Can you work these out from the model? Positions are in its coordinate system, mm. Round coordinates to 2 decimals unless told otherwise and drop trailing zeros. Order: outer loops, then holes, each group sorted by start corner. A loop starts at its lowest first (then second) coordinate and runs counter-clockwise, first axis right, second up. Notation, with made-up numbers: (17.5, 3.25) - (34.5, 3.25) arc R22 ccw to (34.5, 11.25) - close; hole circle Ø10 at (30, 70). An arc over 180 degrees is marked (long way). Write item = value, one per line.
from build123d import *

# Parameters (mm, degrees)
BOSS_EXTRUDE1_DEPTH = 2
SKETCH2_W           = 40
SKETCH2_H           = 13
BOSS_EXTRUDE2_DEPTH = 2.8


with BuildPart() as part:
    # Sketch1 → Boss-Extrude1 (new body)
    with BuildSketch(Plane.XY):
        Polygon((-9.9, -17.9), (-4, -17.9), (-4, -16.4), (4, -16.4), (4, -17.9), (9.9, -17.9), (9.9, -10.1), (27.9, -10.1), (27.9, 10.7), (20.7, 10.7), (20.7, 17.9), (-20.7, 17.9), (-20.7, 10.7), (-27.9, 10.7), (-27.9, -10.1), (-9.9, -10.1), align=None)
    extrude(amount=-BOSS_EXTRUDE1_DEPTH)

    # Sketch2 → Boss-Extrude2 (add)
    with BuildSketch(Plane(origin=(0, 0, -2), x_dir=(-1, 0, 0), z_dir=(0, 0, -1))):
        with Locations((0, -1.7)):
            Rectangle(SKETCH2_W, SKETCH2_H)
    extrude(amount=BOSS_EXTRUDE2_DEPTH)


solid = part.part
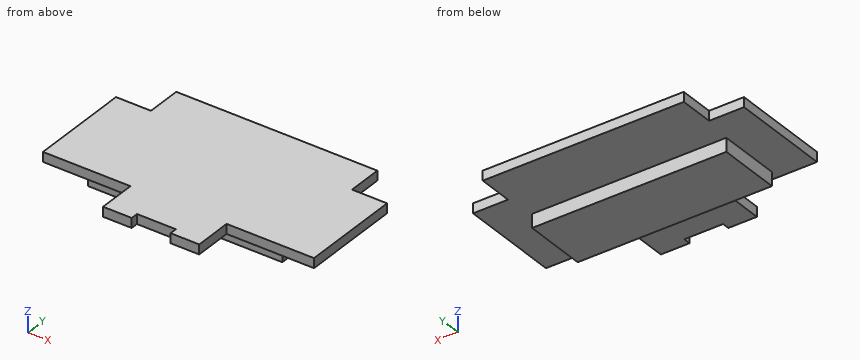
(1) If we section it at B-B (z = -1.15): Write out the boundary of the cut face in (x, y), plus the area to 3 significant figures.
Computed:
outline = (-27.9, -10.1) - (-9.9, -10.1) - (-9.9, -17.9) - (-4, -17.9) - (-4, -16.4) - (4, -16.4) - (4, -17.9) - (9.9, -17.9) - (9.9, -10.1) - (27.9, -10.1) - (27.9, 10.7) - (20.7, 10.7) - (20.7, 17.9) - (-20.7, 17.9) - (-20.7, 10.7) - (-27.9, 10.7) - close
area = 1,600 mm^2
(2) If we section it at C-C (y = 3): Write out the boundary of the cut face in (x, z).
Computed:
outline = (-27.9, -2) - (-20, -2) - (-20, -4.8) - (20, -4.8) - (20, -2) - (27.9, -2) - (27.9, 0) - (-27.9, 0) - close
(3) Will these pins go through, and if not, where does the flat tip stop? P1, Ø1.6, axis at x = 23, z = -1.5, coming from the +Y side; P2, Ø1.6, axis at y = -17.5, z = -1, coming from the -X side; P3, Ø1.6, axis at y = -13.5, z = -0.5, coming from the +X side.
Computed:
P1 = 10.7
P2 = -9.9
P3 = 9.9
(4) If we section it at D-D (y = 8.5): Write out the boundary of the cut face in (x, z).
Computed:
outline = (-27.9, -2) - (27.9, -2) - (27.9, 0) - (-27.9, 0) - close
(5) If we section it at A-A (x = -11.5): Write out the boundary of the cut face in (y, z).
Computed:
outline = (-10.1, -2) - (-8.2, -2) - (-8.2, -4.8) - (4.8, -4.8) - (4.8, -2) - (17.9, -2) - (17.9, 0) - (-10.1, 0) - close
(6) If I drill on line 1 (Y direction, x = 3, z = -1.3); line 2 (X direction, y = 12, z = -1.3); line 3 (Y direction, x = 7, z = -3.15), over which ranges is the centre line in solid material (lowest first)? Write a range as from..to.
Computed:
line_1 = -16.4..17.9
line_2 = -20.7..20.7
line_3 = -8.2..4.8
